Part model, mm, in its own coordinate system. A direction names the side the tool comes from. Round coordinates to 2 decimals unless told otherwise and drop trailing zeros. Loops run counter-clockwise (first coordinate to the right, second up) from the corner with the lowest first, then second, coordinate; pieces in that order, holes last. Notation, with made-up numbers: (41.5, 22) - (52.5, 22) arc R6 ccw to (52.5, 27) - close; hole circle Ø4 at (74, 89). An arc over 180 degrees is marked (long way). Put each result on its own line as item: value.
Autodesk Inventor part; units mm, degrees
ref_plane "Work Plane1" through (-276, 67.1224, -42.5) normal (0, -1, 0) x (1, 0, 0)
ref_plane "YZ Plane" through (0, 0, 0) normal (1, 0, 0) x (0, 1, 0)
ref_plane "XZ Plane" through (0, 0, 0) normal (0, 1, 0) x (-1, 0, 0)
sketch "Sketch1" plane through (0, 0, 0) normal (1, 0, 0) x (0, 1, 0)
  line L0 (0, 0) -> (440, 0)
  line L1 (440, 0) -> (440, -100)
  line L2 (440, -100) -> (0, -100)
  line L3 (0, -100) -> (0, 0)
  line L4 (0, 0) -> (0, 23.0594)
  line L5 (0, 23.0594) -> (440, 0)
  dimension "d0" = 100
  dimension "d1" = 87
  dimension "d32" = 440
extrude "top" add sketch "Sketch1" along normal mid plane 25
sketch "Sketch2" plane through (0, 0, 0) normal (1, 0, 0) x (0, 1, 0)
  line L0 (0, -100) -> (440, -100)
  line L1 (0, -100) -> (-20, -100)
  line L2 (-20, -100) -> (-20, 100)
  line L3 (-20, 100) -> (0, 100)
  line L4 (0, 100) -> (0, -100)
  point P0 (0, 0)
  dimension "d4" = 20
  dimension "d9" = 200
extrude "bott" add sketch "Sketch2" along normal mid plane 85
sketch "Sketch4" plane through (-12.5, 0, 0) normal (-1, 0, 0) x (0, 0, 1)
  line L0 (0, 440) -> (-100, 440)
  line L1 (-100, 0) -> (23.0594, 0)
  line L2 (-100, 440) -> (-70, 440)
  line L3 (-70, 440) -> (-70, 0)
  line L4 (-70, 0) -> (-100, 0)
  line L5 (-100, 0) -> (-100, 440)
  point P0 (0, 0)
  dimension "d11" = 30
extrude "arm" add sketch "Sketch4" along normal blind 30
sketch "Sketch5" plane through (42.5, -20, -100) normal (0, 0, -1) x (-1, 0, 0)
  line L0 (0, 0) -> (0, 20)
  line L1 (85, 0) -> (0, 0)
  line L2 (0, 20) -> (85, 20)
  line L3 (85, 20) -> (85, 0)
  line L4 (85, 0) -> (0, 0)
  line L5 (0, 0) -> (0, 20)
  point P0 (42.5, 20)
extrude "back" add sketch "Sketch5" along normal blind 80
sketch "Sketch8" plane through (-12.5, 440, 0) normal (0, 1, 0) x (1, 0, 0)
  line L0 (25, 0) -> (0, 0) construction
  line L1 (25, 100) -> (25, 0) construction
  line L2 (-30, 100) -> (25, 100) construction
  line L3 (-30, 70) -> (-30, 100) construction
  line L4 (0, 70) -> (-30, 70) construction
  line L5 (0, 0) -> (0, 70) construction
  line L6 (0, 71.4142) -> (-1.4142, 70)
  line L7 (-1.4142, 70) -> (0, 68.5858)
  line L8 (0, 68.5858) -> (1.4142, 70)
  line L9 (1.4142, 70) -> (0, 71.4142)
  line L10 (0, 71.4142) -> (0, 68.5858) construction
  line L11 (-1.4142, 70) -> (1.4142, 70) construction
  point P0 (12.5, 0)
  point P1 (0, 70)
  dimension "d33" = 2
  dimension "d34" = 2
ref_plane "Work Plane1" through (-276, 67.1224, -42.5) normal (0, -1, 0) x (1, 0, 0)
extrude "Extrusion7" cut sketch "Sketch8" against normal up to surface (372.8776 mm away)
sketch "Sketch9" plane through (12.5, 0, -100) normal (0, 0, -1) x (-1, 0, 0)
  circle A0 centre (331, 90) radius 5.25 construction
  circle A1 centre (331, 170) radius 5.25 construction
  circle A2 centre (331, 250) radius 5.25 construction
  circle A3 centre (331, 330) radius 5.25 construction
  circle A4 centre (331, 410) radius 5.25 construction
  circle A5 centre (39, 90) radius 5.25 construction
  circle A6 centre (39, 170) radius 5.25 construction
  circle A7 centre (39, 250) radius 5.25 construction
  circle A8 centre (39, 330) radius 5.25 construction
  circle A9 centre (39, 410) radius 5.25 construction
  circle A10 centre (147.5, 100) radius 2.567 construction
  circle A11 centre (222.5, 100) radius 2.567 construction
  circle A12 centre (147.5, 200) radius 2.567 construction
  circle A13 centre (222.5, 200) radius 2.567 construction
  circle A14 centre (147.5, 300) radius 2.567 construction
  circle A15 centre (222.5, 300) radius 2.567 construction
  circle A16 centre (147.5, 400) radius 2.567 construction
  circle A17 centre (222.5, 400) radius 2.567 construction
  line L0 (25, 60) -> (25, 440) construction
  line L1 (345, 60) -> (25, 60) construction
  line L2 (345, 440) -> (345, 60) construction
  line L3 (25, 440) -> (345, 440) construction
hole "Hole2" at (-26.5, 410, -100) at (-26.5, 330, -100) at (-26.5, 250, -100) at (-26.5, 170, -100) at (-26.5, 90, -100) direction (0, 0, 1) diameter 8.376 depth 30
chamfer "Chamfer4" distance 0.5 angle 45 5 edges at (-26.5, 325.812, -70) (-26.5, 405.812, -70) (-26.5, 85.812, -70) (-26.5, 165.812, -70) (-26.5, 245.812, -70)
mirror "Mirror1" about plane through (0, 0, 0) normal (1, 0, 0) of "arm", "Hole2", "Chamfer4"
fillet "Fillet1" radius 10 6 edges at (27.5, 0, -70) (12.5, 0, -23.4703) (0, 0, 23.0594) (-12.5, 0, -23.4703) (-27.5, 0, -70) (0, 0, -100)
sketch "Sketch10" plane through (-42.5, 0, 100) normal (0, 1, 0) x (1, 0, 0)
  line L0 (42.5, 336) -> (42.5, -56)
  line L1 (85, 0) -> (0, 0)
  line L2 (0, 280) -> (85, 280)
  point P0 (42.5, 100)
  point P1 (17.5, 20)
  point P2 (67.5, 20)
  point P3 (67.5, 50)
  point P4 (17.5, 50)
  point P5 (67.5, 260)
  point P6 (17.5, 260)
  point P7 (67.5, 230)
  point P8 (17.5, 230)
  dimension "d51" = 50
  dimension "d52" = 20
  dimension "d53" = 30
  dimension "d54" = 20
  dimension "d55" = 30
hole "Hole3" at (-25, 0, 80) at (25, 0, 80) at (25, 0, 50) at (-25, 0, 50) at (25, 0, -160) at (-25, 0, -160) at (25, 0, -130) at (-25, 0, -130) direction (0, -1, 0) diameter 10.5 end through all
chamfer "Chamfer5" distance 0.5 angle 45 4 edges at (-25, 0, 44.75) (25, 0, 44.75) (-25, 0, 74.75) (25, 0, 74.75)
properties part number "KN-00-01-04" material "X5CrNi18-10"
1. Tool access for faces 1 (the flat face through (27, 222, -70)), 2 (the cylindrical face through (23.4, -10.1, -125)), 3 (the flat face through (1, 0, -145)): list every direction of +Z, -Z, +X, -X, +Y, -Y with a clear straight run to the whole face (end or side of a thin tool).
A:
face 1: +Z, +X, +Y
face 2: +Y, -Y
face 3: -Z, +X, -X, +Y
2. Band-saw the part on C-C (z = -36.5). List the corners of the cut face in (x, y).
A:
outline: (-42.5, -20) - (42.5, -20) - (42.5, 0) - (22.5, 0) arc R10 cw to (12.5, 10) - (12.5, 440) - (-12.5, 440) - (-12.5, 10) arc R10 cw to (-22.5, 0) - (-42.5, 0) - close
3. Band-saw the part on A-A (z = -130). List the corners of the cut face in (x, y).
A:
outline: (-42.5, -20) - (-30.25, -20) - (-30.25, 0) - (-42.5, 0) - close; (-19.75, -20) - (19.75, -20) - (19.75, 0) - (-19.75, 0) - close; (30.25, -20) - (42.5, -20) - (42.5, 0) - (30.25, 0) - close
4. Band-saw the part on B-B (y = 309). List the corners of the cut face in (x, z).
A:
outline: (-42.5, -100) - (42.5, -100) - (42.5, -70) - (12.5, -70) - (12.5, 6.87) - (-12.5, 6.87) - (-12.5, -68.59) - (-11.09, -70) - (-12.5, -71.41) - (-13.91, -70) - (-42.5, -70) - close
5. Pin check, flat tips, straight feed: P1, Ø6.5, axis at x = 25, z = 80, coming from the +Y side; P2, Ø9.5, axis at x = 26.5, y = 90, coming from the +Z side; P3, Ø0.8, axis at x = -12.5, z = -70.5, coming from the +Y side; P4, Ø10, axis at x = 18.5, y = 202.5, coming from the -Z side. Stop position of each tip, or through.
A:
P1: passes through
P2: stops at z = -70
P3: stops at y = 67.12
P4: stops at z = -100
6. Two-plate mould, pull along Y, no slides. Class faces 4 (the cylindrical face through (-26.684, 245.816, -85.044)), 5 (the flat face through (-1, 440, -62)), 6 (the cylindrical face through (-26.684, 165.816, -85.044)), 7 (the cylindrical face through (-21.81, -10.39, 45.83)): pulls with the +Y half, pulls with the -Y half, needs draft (parallel to the pull), parting line crosses it, or undercut.
A:
face 4: undercut
face 5: pulls with the +Y half
face 6: undercut
face 7: needs draft
7. Probe line 1 along Y through (x, z) = (-26.5, -83); line 2 along Z through (x, y) = (25, -4.25); line 3 along X through (y, z) = (-9, -160). List the from-to ranges inside material, lowest first. Write a range as [from, to].
A:
line 1: y = [-20, 85.81], [94.19, 165.81], [174.19, 245.81], [254.19, 325.81], [334.19, 405.81], [414.19, 440]
line 2: z = [-180, -165.25], [-154.75, -135.25], [-124.75, 44.75], [55.25, 74.75], [85.25, 100]
line 3: x = [-42.5, -30.25], [-19.75, 19.75], [30.25, 42.5]
8. Band-saw the part on D-D (y = 378.5). List the corners of the cut face in (x, z).
A:
outline: (-42.5, -100) - (42.5, -100) - (42.5, -70) - (12.5, -70) - (12.5, 3.22) - (-12.5, 3.22) - (-12.5, -68.59) - (-11.09, -70) - (-12.5, -71.41) - (-13.91, -70) - (-42.5, -70) - close
